Here's how the part is built. I have some questions about the finished solid (model axes, mm). A direction names the side the tool comes from. Coordinates: 2 decimals unless noted, no trailing zeros. Write each loop counter-clockwise with the first axis right and the second up, starting at its lowest first coordinate (ties: lowest second). Pieces come first, ordered by that corner, then holes.
Autodesk Inventor part; units mm, degrees
ref_plane "YZ Plane" through (0, 0, 0) normal (1, 0, 0) x (0, 1, 0)
ref_plane "XZ Plane" through (0, 0, 0) normal (0, 1, 0) x (-1, 0, 0)
ref_plane "XY Plane" through (0, 0, 0) normal (0, 0, 1) x (1, 0, 0)
sketch "Sketch1" plane through (0, 0, 0) normal (0, 0, 1) x (1, 0, 0)
  line L0 (-17.78, 0) -> (17.78, 0)
  line L1 (0, -17.78) -> (0, 17.78)
  line L2 (-12.7, 12.7) -> (12.7, 12.7)
  line L3 (12.7, 12.7) -> (12.7, -12.7)
  line L4 (12.7, -12.7) -> (-12.7, -12.7)
  line L5 (-12.7, -12.7) -> (-12.7, 12.7)
  line L6 (9.525, 9.525) -> (-9.525, 9.525)
  line L7 (-9.525, 9.525) -> (-9.525, -9.525)
  line L8 (-9.525, -9.525) -> (9.525, -9.525)
  line L9 (9.525, -9.525) -> (9.525, 9.525)
  point P0 (0, 0)
  point P1 (-12.7, 0)
  point P2 (0, 12.7)
  dimension "d0" = 25.4
  dimension "d1" = 3.175
extrude "Extrusion1" add sketch "Sketch1" along normal mid plane 457.2 contours L5 L2 L1 L6 L7 L0 | L0 L7 L8 L1 L4 L5 | L1 L8 L9 L0 L3 L4 | L2 L3 L0 L9 L6 L1
sketch "Sketch3" plane through (-12.7, 12.7, 228.6) normal (0, 1, 0) x (1, 0, 0)
  line L0 (0, 0) -> (25.4, 0)
  line L1 (25.4, 0) -> (25.4, 457.2)
  line L2 (0, 457.2) -> (0, 0)
  line L3 (0, 0) -> (25.4, 19.4901)
  line L4 (0, 228.6) -> (25.4, 228.6) construction
  line L5 (0, 0) -> (25.4, 0)
  line L6 (25.4, 0) -> (25.4, 19.4901)
  line L7 (0, 457.2) -> (25.4, 437.7099)
  line L8 (0, 457.2) -> (25.4, 457.2)
  line L9 (25.4, 457.2) -> (25.4, 437.7099)
  point P0 (12.7, 228.6)
  dimension "d7" = 37.5
extrude "Extrusion3" cut sketch "Sketch3" against normal through all contours L3 L1 L0 | L8 L1 L7
properties part number "tubing_template_0.125" material "Aluminum-6061"
1) Imagine slicing it at A-A on y = -3.5. Please give me the cut outline in (x, z) (3 decimals), then the cut area to 3 significant figures.
Values follow:
outline: (-12.7, -228.6) - (-9.525, -226.164) - (-9.525, 226.164) - (-12.7, 228.6) - close; (9.525, -211.546) - (12.7, -209.11) - (12.7, 209.11) - (9.525, 211.546) - close
area: 2,780 mm2
2) I need wall thicknesses on probe 1 along Y at (x, z) = (6, 59.5) (3 decimals); probe 2 along Z at (x, y) = (-11.25, 1). Which ranges of each line are inside material? Lowest first, please.
Values follow:
probe 1: y = -12.7 to -9.525, 9.525 to 12.7
probe 2: z = -227.49 to 227.49
3) Imagine slicing it at B-B on z = 84.5. Please give me the cut outline in (x, y) (3 decimals).
Values follow:
outline: (-12.7, -12.7) - (12.7, -12.7) - (12.7, 12.7) - (-12.7, 12.7) - close; hole (-9.525, -9.525) - (9.525, -9.525) - (9.525, 9.525) - (-9.525, 9.525) - close
4) On a 3-axis mill with a long thin cutter (end or side, diameter ignored), from which of +Z, -Z, +X, -X, +Y, -Y can I reach the whole of each face in a straight line? I mean faces 5 (the face through (0, 9.525, -3)), 6 (the face through (-12.7, 0, -3)). Say none if no direction works.
Values follow:
face 5: +Z, -Z
face 6: +Z, -Z, -X, +Y, -Y
5) We'd pull the mould along X, two halves only. Please class faces 1 (the face through (0, -9.525, -3)), 2 (the face through (12.7, 0, -3)), 3 (the face through (0, -12.7, -3)), 4 (the face through (9.525, 0, -3)): pulls with the +X half, pulls with the -X half, needs draft (parallel to the pull), parting line crosses it, or undercut.
Values follow:
face 1: undercut
face 2: pulls with the +X half
face 3: needs draft
face 4: undercut
6) Imagine slicing it at C-C on x = -2.25. Please give me the cut outline in (y, z) (3 decimals).
Values follow:
outline: (-12.7, -220.581) - (-9.525, -220.581) - (-9.525, 220.581) - (-12.7, 220.581) - close; (9.525, -220.581) - (12.7, -220.581) - (12.7, 220.581) - (9.525, 220.581) - close
